Check sheet for the modelled part. Datum: model origin and axes. Units: mm. Give positions to 0.01 mm unless a question says otherwise; leave off trailing zeros. Order: outer loops, then holes, each group sorted by start corner. A loop starts at its lowest first (then second) coordinate and runs counter-clockwise, first axis right, second up. Notation, with made-up numbers: (79, 6.25) -> (120, 6.25) arc R13 cw to (120, 23.25) -> close; hole circle Ø4 at (24.5, 20). An arc over 180 degrees is marked (long way). Answer in a Markdown table with one row per item. Add a question column.
(1) Go/stop test with flat-tipped pins: pin 1 (4 mm diameter, centred on x = -30, z = 17.5, fed in from -Y); pin 2 (2.5 mm diameter, centred on x = -14, z = 0, fed in from -Y); pin 3 (2 mm diameter, centred on x = -26, z = 14.5, fed in from +Y); pin 4 (1.6 mm diameter, centred on x = -29, y = 0.5, fed in from -Z). Record where each tip stops, or that it passes through.
(2) Cross-section at B-B (x = -30). State how many separate pieces and enclosed holes the cut face has, then the cut area to 3 significant figures.
(3) Release check for a two-part mould opening along X. For faces 1 (the face through (0, 4, -1)), 2 (the face through (-17, 1.5, -1)), 3 (the face through (16.464, 3.131, -0.325)) record: released by +X, released by -X, zero draft, split by the parting line, or undercut.
(4) Thickness scan on L1, parallel to Z at x = -14, y = 0.6; L2, parallel to Z at x = 15, y = 3; L3, parallel to X at y = 2.25, z = 35. Record the ranges inside material, lowest first. Write a range as [from, to].
(5) Cross-section at A-A (z = 35). Record the cut outline in (x, y), then the cut area to 3 significant figures.
(6) Cross-section at C-C (y = 4). Record the cut outline in (x, z).
(7) Cross-section at D-D (x = -14). Record the cut outline in (y, z), then the cut area to 4 significant figures.
Autodesk Inventor part; units mm, degrees
ref_plane "YZ Plane" through (0, 0, 0) normal (1, 0, 0) x (0, 1, 0)
ref_plane "XZ Plane" through (0, 0, 0) normal (0, 1, 0) x (-1, 0, 0)
ref_plane "XY Plane" through (0, 0, 0) normal (0, 0, 1) x (1, 0, 0)
sketch "Esboço1" plane through (0, 0, 0) normal (0, 1, 0) x (-1, 0, 0)
  line L0 (-35, -50) -> (35, -50)
  line L1 (35, -50) -> (35, 50)
  line L2 (35, 50) -> (-35, 50)
  line L3 (-35, 50) -> (-35, -50)
  line L4 (-35, -50) -> (35, 50) construction
  line L5 (35, -50) -> (-35, 50) construction
  point P0 (0, 0)
  dimension "d0" = 70
  dimension "d1" = 100
extrude "Extrusão1" add sketch "Esboço1" along normal blind 6.35
sketch "Esboço2" plane through (35, 0, -50) normal (0, 0, -1) x (-1, 0, 0)
  line L0 (10, 6.35) -> (0, 1.3533)
  line L1 (0, 1.3533) -> (37.5, 1.3533) construction
  line L2 (0, 0) -> (0, 6.35)
  line L3 (0, 6.35) -> (70, 6.35)
  line L4 (0, 0) -> (70, 0)
  line L5 (70, 0) -> (70, 6.35)
  line L6 (0, 6.35) -> (70, 6.35)
  line L7 (0, 0) -> (0, 6.35)
  line L8 (10, 6.35) -> (35, 6.35)
  line L9 (70, 6.35) -> (0, 6.35)
  line L10 (35, 6.35) -> (35, 1.5)
  line L11 (35, 1.5) -> (70, 1.5)
  line L12 (70, 0) -> (70, 6.35)
  point P0 (35, 0)
  point P1 (70, 1.5)
  point P2 (35, 6.35)
  dimension "d7" = 25
  dimension "d8" = 26.55
  dimension "d9" = 1.5
  dimension "d16" = 35
extrude "Extrusão2" cut sketch "Esboço2" against normal through all contours L0 L2 L3 | L3 L5 L11 L10
sketch "Esboço3" plane through (-35, 1.5, -50) normal (0, 1, 0) x (1, 0, 0)
  line L0 (0, -77.5) -> (10, -77.5)
  line L1 (10, -77.5) -> (10, -22.5)
  line L2 (10, -22.5) -> (0, -22.5)
  line L3 (0, -22.5) -> (0, -77.5)
  line L4 (0, -77.5) -> (10, -22.5) construction
  line L5 (10, -77.5) -> (0, -22.5) construction
  line L6 (0, -100) -> (0, 0)
  line L7 (35, -100) -> (0, -100)
  line L8 (35, 0) -> (35, -100)
  line L9 (0, 0) -> (35, 0)
  line L10 (0, -100) -> (0, 0)
  line L11 (10, -77.5) -> (10, -100)
  line L12 (0, -100) -> (70, -100)
  line L13 (10, -22.5) -> (10, 0)
  line L14 (70, 0) -> (0, 0)
  point P0 (35, -50)
  point P1 (5, -50)
  point P2 (5, -50)
  point P3 (10, -100)
  dimension "d12" = 10
  dimension "d13" = 55
extrude "Extrusão3" cut sketch "Esboço3" against normal through all contours L0 L11 L7 L6 | L6 L9 L13 L2
sketch "Esboço10" plane through (0, 1.5, 50) normal (0, 1, 0) x (1, 0, 0)
  line L0 (-35, 22.5) -> (-25, 22.5)
  line L1 (-25, 77.5) -> (-35, 77.5)
  line L2 (0, 0) -> (-25, 0)
  line L3 (-25, 22.5) -> (-25, 0)
  point P0 (0, 50)
  point P1 (-30, 32.5)
  point P2 (-30, 50)
  point P3 (-30, 67.5)
  dimension "d61" = 10
  dimension "d62" = 10
  dimension "d63" = 50
  dimension "d64" = 5
hole "Furo3" at (-30, 1.5, 17.5) at (-30, 1.5, 0) at (-30, 1.5, -17.5) direction (0, -1, 0) diameter 3 end through all
chamfer "Chanfro1" distance 1.5 angle 45 3 edges at (-30, 0, -19) (-30, 0, -1.5) (-30, 0, 16)
sketch "Esboço11" plane through (0, 6.35, 0) normal (0, 1, 0) x (1, 0, 0)
  line L0 (0, 50) -> (0, -50)
  line L1 (25, -50) -> (25, 50)
  point P0 (0, 0)
  point P1 (15, -35)
  point P2 (15, 0)
  point P3 (15, 35)
  point P4 (0, 0)
  point P5 (-14, 0)
  point P6 (-14, -43)
  point P7 (-14, 43)
  dimension "d75" = 10
  dimension "d76" = 35
  dimension "d77" = 35
  dimension "d78" = 29
  dimension "d79" = 43
  dimension "d80" = 43
hole "Furo4" at (15, 6.35, 35) at (15, 6.35, 0) at (15, 6.35, -35) at (-14, 6.35, 0) at (-14, 6.35, 43) at (-14, 6.35, -43) direction (0, -1, 0) diameter 3 end through all
properties part number "Base Aço" material "Aço"
Answer below:
| question | item | result |
|---|---|---|
| 1 | pin 1 | stops at y = 1 |
| 1 | pin 2 | passes through |
| 1 | pin 3 | stops at y = 1.5 |
| 1 | pin 4 | stops at z = -27.5 |
| 2 | separate pieces | 4 |
| 2 | enclosed holes | 0 |
| 2 | area | 62.3 mm² |
| 3 | face 1 | released by -X |
| 3 | face 2 | zero draft |
| 3 | face 3 | undercut |
| 4 | L1 | z = [-50, -44.5], [-41.5, -1.5], [1.5, 41.5], [44.5, 50] |
| 4 | L2 | z = [-50, -36.5], [-33.5, -1.5], [1.5, 33.5], [36.5, 50] |
| 4 | L3 | x = [0, 13.5], [16.5, 33.21] |
| 5 | outline | (-25, 0) -> (13.5, 0) -> (13.5, 6.35) -> (0, 6.35) -> (0, 1.5) -> (-25, 1.5) -> close; (16.5, 0) -> (35, 0) -> (35, 1.35) -> (25, 6.35) -> (16.5, 6.35) -> close |
| 5 | area | 216 mm² |
| 6 | outline | (0, -50) -> (29.7, -50) -> (29.7, 50) -> (0, 50) -> close; hole circle Ø3 at (15, -35); hole circle Ø3 at (15, 0); hole circle Ø3 at (15, 35) |
| 7 | outline | (0, -50) -> (1.5, -50) -> (1.5, -44.5) -> (0, -44.5) -> close; (0, -41.5) -> (1.5, -41.5) -> (1.5, -1.5) -> (0, -1.5) -> close; (0, 1.5) -> (1.5, 1.5) -> (1.5, 41.5) -> (0, 41.5) -> close; (0, 44.5) -> (1.5, 44.5) -> (1.5, 50) -> (0, 50) -> close |
| 7 | area | 136.5 mm² |
